```python
from build123d import *

# Parameters (mm, degrees)
F1_W     = 26
F1_H     = 40
F2_DEPTH = 7
F0_W     = 40
F0_H     = 19
F3_DEPTH = 3.5


with BuildPart() as f2:
    # F1 (on Top) → F2 (new body)
    with BuildSketch(Plane.XY):
        Rectangle(F1_W, F1_H)
    extrude(amount=F2_DEPTH)

    # F0 (on Right) → F3 (join, symmetric)
    with BuildSketch(Plane.YZ):
        with Locations((-0.3058470263, -9.5)):
            Rectangle(F0_W, F0_H)
    extrude(amount=F3_DEPTH, both=True)


solid = f2.part
```
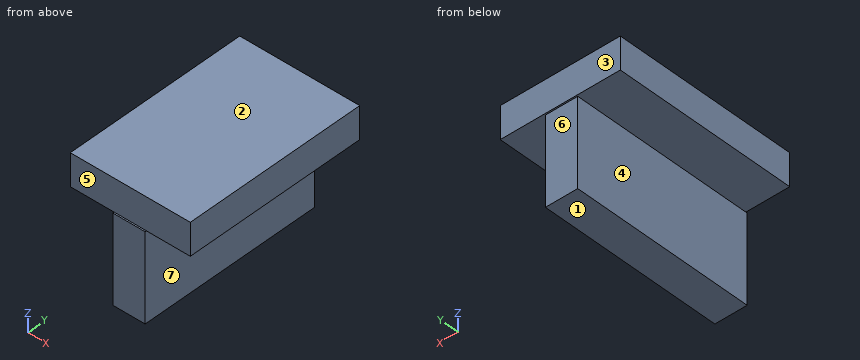
For this review, take the finished solid that the model builds, in its own axes (mm). Face numbers are marked on the shaded views. A direction names the side the tool comes from. Round coordinates to 2 decimals unless told otherwise and drop trailing zeros. Order: outer loops, then holes, each group sorted by start corner. A loop starts at its lowest first (then second) coordinate and runs counter-clockwise, first axis right, second up. Notation, with made-up numbers: (-24.5, 35.5) -> (-16.5, 35.5) arc R13 cw to (-16.5, 51.5) -> close; hole circle Ø3 at (-13.5, 65). An arc over 180 degrees is marked (long way). Use a Markdown table: item, result.
Item 1: Take a section at C-C (z = -4.5). State the section outline as (x, y) points.
Resolved:
| item | result |
|---|---|
| outline | (-3.5, -20.31) -> (3.5, -20.31) -> (3.5, 19.69) -> (-3.5, 19.69) -> close |
Item 2: For pin 1 (12 mm diameter, centred on x = -1.5, z = -16, fed in from +Y); pin 2 (3 mm diameter, centred on x = -8.5, z = 1.5, fed in from -Y); pin 3 (5.5 mm diameter, centred on y = 0.5, z = -5, fed in from -X), all flat-tipped, find the tip position at first contact; note any pin that passes through.
Resolved:
| item | result |
|---|---|
| pin 1 | stops at y = 19.69 |
| pin 2 | stops at y = -20 |
| pin 3 | stops at x = -3.5 |
Item 3: Draft analysis for pull direction Z (two halves, no side actions). For the marked faces 1, 2 and 3, state which applies: +Z half, -Z half, draft (parallel to the pull), parting line (faces both ways), or undercut.
Resolved:
| item | result |
|---|---|
| face 1 | -Z half |
| face 2 | +Z half |
| face 3 | draft |
Item 4: For line 1 along X through (y, z) = (-11.5, -5.75); line 2 along Z through (x, y) = (10.25, -1.5); line 3 along Y through (x, z) = (-4, 5), list the stretches that pass through material, from the lowest coordinate up. Write a range as [from, to].
Resolved:
| item | result |
|---|---|
| line 1 | x = [-3.5, 3.5] |
| line 2 | z = [0, 7] |
| line 3 | y = [-20, 20] |
Item 5: Take a section at A-A (y = -3.5). State the section outline as (x, z) points.
Resolved:
| item | result |
|---|---|
| outline | (-13, 0) -> (-3.5, 0) -> (-3.5, -19) -> (3.5, -19) -> (3.5, 0) -> (13, 0) -> (13, 7) -> (-13, 7) -> close |
Item 6: Machinability: for the marked faces 4, 5, 6 and 7, which of the approach directions +Z, -Z, +X, -X, +Y, -Y give a long, thin tool a straight path to every point of the face, cutting with its end or side? Answer none if there is none.
Resolved:
| item | result |
|---|---|
| face 4 | -Z, -X, +Y, -Y |
| face 5 | +Z, +X, -X, -Y |
| face 6 | -Z, +X, -X, +Y |
| face 7 | -Z, +X, +Y, -Y |
Item 7: Take a section at B-B (x = 8.5). State the section outline as (y, z) points, plus the area to 3 significant figures.
Resolved:
| item | result |
|---|---|
| outline | (-20, 0) -> (20, 0) -> (20, 7) -> (-20, 7) -> close |
| area | 280 mm² |
